Source: three-view drawing plus pictorial views. Frame: mm from the lowest corner of the part. A direction names the side the tool comes from. Round coordinates to 2 decimals unless told otherwise and drop trailing zeros. Write each loop counter-clockwise with the first axis right and the second up, starting at its lowest first coordinate (ties: lowest second). Pieces come first, ordered by that corner, then holes. Notation, with made-up numbers: (44, -16) - (67, -16) arc R18 ccw to (67, 18) - close; hole circle Ø8 at (44, 63). An arc over 180 degrees is marked (long way). Write each question's results on one line, items separated by ' | '.
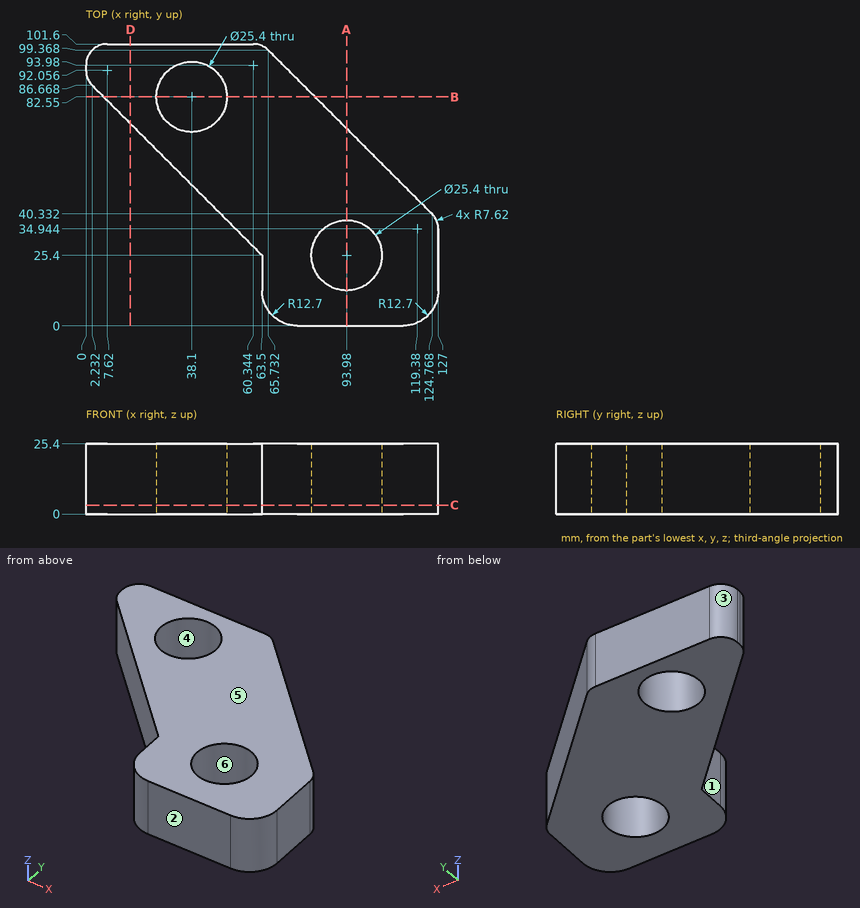
Q1. Ray query, line 1 along Y through (x, z) = (38.1, 19.75); line 2 along X through (y, z) = (24, 3); line 3 along X through (y, z) = (34, 10) (1 decimal). Return the intervals inside material, ascending.
Answer block:
line 1: 50.8 to 69.85, 95.25 to 101.6 | line 2: 63.5 to 81.36, 106.6 to 127 | line 3: 54.9 to 84.6, 103.3 to 127
Q2. Pin query (flat end, axial travel): pin 1 (2 mm diameter, centred on y = 58, z = 21, fed in from -X); pin 2 (6 mm diameter, centred on y = 44.5, z = 15.5, fed in from -X); pin 3 (4 mm diameter, centred on y = 21, z = 13.5, fed in from -X); pin 4 (2 mm diameter, centred on x = 82, z = 13.5, fed in from -Y). Return the tip coordinate at first contact, or that it passes through.
Answer block:
pin 1: x = 29.9 | pin 2: x = 41.4 | pin 3: x = 63.5 | pin 4: y = 0
Q3. Section query B-B, the plane y = 82.55. Return loops of the section in (x, z), plus the area to 3 significant figures.
Answer block:
outline: (6.35, 0) - (25.4, 0) - (25.4, 25.4) - (6.35, 25.4) - close; (50.8, 0) - (82.55, 0) - (82.55, 25.4) - (50.8, 25.4) - close | area: 1,290 mm2
Q4. Section query C-C, the plane z = 3.25. Return loops of the section in (x, y).
Answer block:
outline: (0, 92.06) arc R7.62 ccw to (2.23, 86.67) - (63.5, 25.4) - (63.5, 12.7) arc R12.7 ccw to (76.2, 0) - (114.3, 0) arc R12.7 ccw to (127, 12.7) - (127, 34.94) arc R7.62 ccw to (124.77, 40.33) - (65.73, 99.37) arc R7.62 ccw to (60.34, 101.6) - (7.62, 101.6) arc R7.62 ccw to (0, 93.98) - close; hole circle Ø25.4 at (38.1, 82.55); hole circle Ø25.4 at (93.98, 25.4)
Q5. Mould query, pull axis X, two halves, no side actions, for the marked faces 3, 4, 5 and 6. Classes: pulls with the +X half, pulls with the -X half, needs draft (parallel to the pull), parting line crosses it, or undercut.
Answer block:
face 3: pulls with the -X half | face 4: undercut | face 5: needs draft | face 6: undercut
Q6. Access query for the marked faces 1 and 2. Directions: +Z, -Z, +X, -X, +Y, -Y. A direction counts if a zero-diameter tool reaches every point of the face in a straight line with its end or side. Return the directions, or none.
Answer block:
face 1: +Z, -Z, -X, -Y | face 2: +Z, -Z, +X, -X, -Y
Q7. Section query A-A, the plane x = 93.98. Return loops of the section in (y, z), plus the area to 3 significant figures.
Answer block:
outline: (0, 0) - (12.7, 0) - (12.7, 25.4) - (0, 25.4) - close; (38.1, 0) - (71.12, 0) - (71.12, 25.4) - (38.1, 25.4) - close | area: 1,160 mm2
Q8. Section query D-D, the plane x = 16. Return loops of the section in (y, z), plus the area to 3 significant figures.
Answer block:
outline: (72.9, 0) - (101.6, 0) - (101.6, 25.4) - (72.9, 25.4) - close | area: 729 mm2
